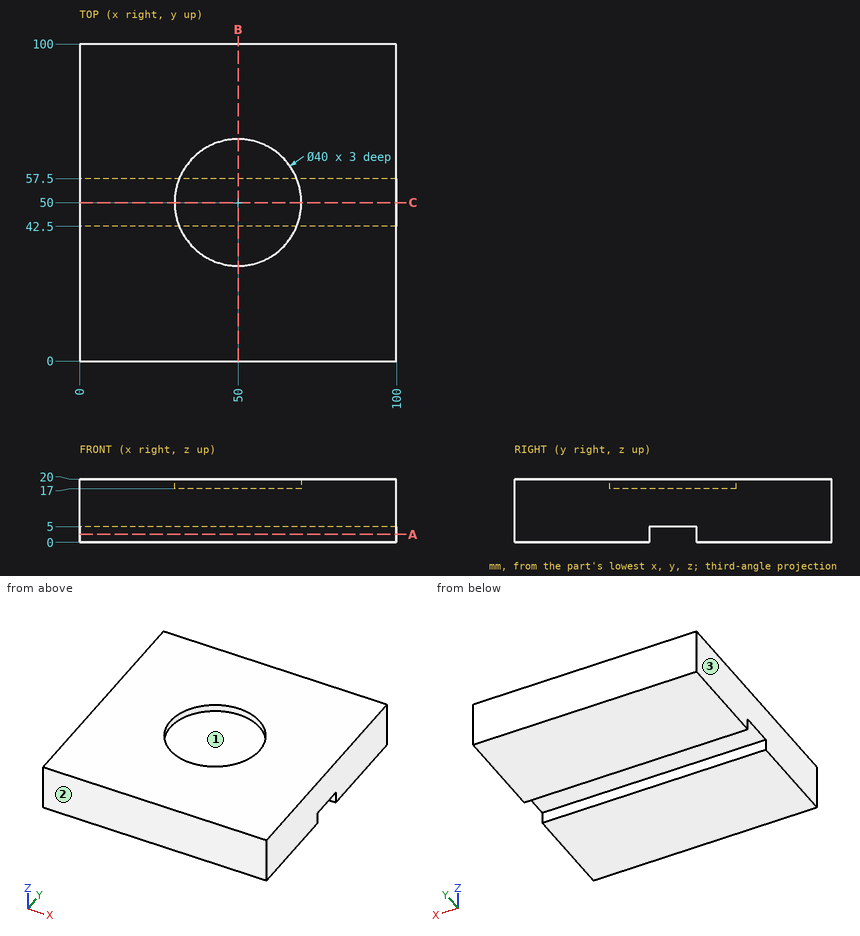
Study the drawing (mm; zero at the part's minimum x, y, z) and answer. Give positions to 0.01 mm unless a question says otherwise; leave off trailing zeros. Write each loop counter-clockwise with the first axis right and the second up, starting at its lowest first coordinate (ties: lowest second). Pieces come first, ordered by that corner, then holes. Notation, with made-up numbers: (-2.75, 47) - (35.25, 47) arc R20 ccw to (35.25, 73) - close; hole circle Ø7 at (50, 65.25). An arc over 180 degrees is marked (long way). Use a Markdown table: item, result.
1. Section B-B on x = 50 is taken. Write down the section's boundary in (y, z), plus the area to 4 significant figures.
Values follow:
| item | result |
|---|---|
| outline | (0, 0) - (42.5, 0) - (42.5, 5) - (57.5, 5) - (57.5, 0) - (100, 0) - (100, 20) - (70, 20) - (70, 17) - (30, 17) - (30, 20) - (0, 20) - close |
| area | 1,805 mm² |
2. Find the intervals of material crossed by probe 1 along Y at (x, z) = (72, 4); probe 2 along Y at (x, z) = (50, 17.95); probe 3 along Z at (x, y) = (21, 50), in increasing order. Write a range as from..to.
Values follow:
| item | result |
|---|---|
| probe 1 | y = 0..42.5, 57.5..100 |
| probe 2 | y = 0..30, 70..100 |
| probe 3 | z = 5..20 |
3. Section C-C on y = 50 is taken. Write down the section's boundary in (x, z).
Values follow:
| item | result |
|---|---|
| outline | (0, 5) - (100, 5) - (100, 20) - (70, 20) - (70, 17) - (30, 17) - (30, 20) - (0, 20) - close |
4. Each of these flat-tipped pins is pushed along its axis until it touches: P1, Ø12, axis at x = 42, y = 52.5, coming from the +Z side; P2, Ø12, axis at y = 66, z = 6.5, coming from the -X side. Where does it stop, or does it pass through?
Values follow:
| item | result |
|---|---|
| P1 | stops at z = 17 |
| P2 | stops at x = 0 |
5. Section A-A on z = 2.5 is taken. Write down the section's boundary in (x, y).
Values follow:
| item | result |
|---|---|
| outline | (0, 0) - (100, 0) - (100, 42.5) - (0, 42.5) - close; (0, 57.5) - (100, 57.5) - (100, 100) - (0, 100) - close |
6. For a pull along X with two mould halves and no side action, classify the marked faces 1, 2 and 3 as released by +X, released by -X, zero draft, split by the parting line, or undercut.
Values follow:
| item | result |
|---|---|
| face 1 | undercut |
| face 2 | zero draft |
| face 3 | released by -X |
